Here's how the part is built. I have some questions about the finished solid (model axes, mm). Face numbers are marked on the shaded views. A direction names the side the tool comes from. Round coordinates to 2 decimals unless told otherwise and drop trailing zeros. Write each loop counter-clockwise with the first axis right and the second up, starting at its lowest first coordinate (ties: lowest second). Pieces come first, ordered by that corner, then holes. Notation, with made-up numbers: (11, 75.5) -> (15, 75.5) arc R25 cw to (15, 102.5) -> close; hole circle Ø10 at (-21.75, 44). An arc over 180 degrees is marked (long way). Answer in a Markdown table with one row per item. Add a question column.
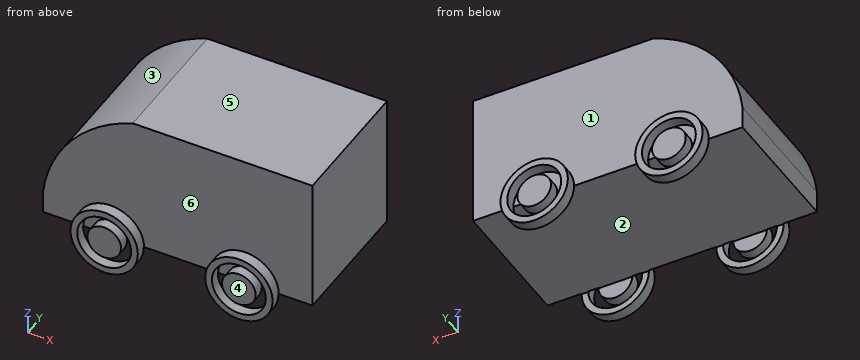
from build123d import *

# Parameters (mm, degrees)
F1_DEPTH = 76.2
F2_R     = 15.24
F3_DEPTH = 6.35
F2_R_2   = 9.525
F4_DEPTH = 6.35
F5_R     = 15.24
F6_DEPTH = 6.35
F5_R_2   = 9.525
F7_DEPTH = 6.35
F8_W     = 152.5372415781
F8_H     = 76.57238096
F9_DEPTH = 25.4


with BuildPart() as f1:
    # F0 (on Front) → F1 (new body)
    with BuildSketch(Plane.XZ):
        with BuildLine():
            Line((82.9111417405, 0), (101.9611417405, 0))
            Line((101.9611417405, 0), (101.9611417405, 76.2))
            Line((101.9611417405, 76.2), (0.3611417405, 76.2))
            ThreePointArc((0.3611417405, 76.2), (-34.2470067394, 51.816518784), (-50.4388582595, 12.7))
            Line((-50.4388582595, 12.7), (-50.4388582595, 0))
            Line((-50.4388582595, 0), (-31.3888582595, 0))
            ThreePointArc((-31.3888582595, 0), (-12.3388582595, 19.05), (6.7111417405, 0))
            Line((6.7111417405, 0), (44.8111417405, 0))
            ThreePointArc((44.8111417405, 0), (63.8611417405, 19.05), (82.9111417405, 0))
        make_face()
        with BuildLine():
            ThreePointArc((44.8111417405, 0), (63.8611417405, -19.05), (82.9111417405, 0))
            Line((82.9111417405, 0), (63.8611417405, 0))
            Line((63.8611417405, 0), (44.8111417405, 0))
        make_face()
        with BuildLine():
            Line((63.8611417405, 0), (82.9111417405, 0))
            ThreePointArc((82.9111417405, 0), (63.8611417405, 19.05), (44.8111417405, 0))
            Line((44.8111417405, 0), (63.8611417405, 0))
        make_face()
        with BuildLine():
            Line((-12.3388582595, 0), (6.7111417405, 0))
            ThreePointArc((6.7111417405, 0), (-12.3388582595, 19.05), (-31.3888582595, 0))
            Line((-31.3888582595, 0), (-12.3388582595, 0))
        make_face()
        with BuildLine():
            ThreePointArc((-31.3888582595, 0), (-12.3388582595, -19.05), (6.7111417405, 0))
            Line((6.7111417405, 0), (-12.3388582595, 0))
            Line((-12.3388582595, 0), (-31.3888582595, 0))
        make_face()
    extrude(amount=F1_DEPTH)

    # F2 (on face) → F3 (join)
    with BuildSketch(Plane.XZ.offset(76.2)):
        with BuildLine():
            ThreePointArc((82.9111417405, 0), (63.8611417405, 19.05), (44.8111417405, 0))
            ThreePointArc((44.8111417405, 0), (63.8611417405, -19.05), (82.9111417405, 0))
        make_face()
        with Locations((63.8611417405, 0)):
            Circle(F2_R, mode=Mode.SUBTRACT)
        with BuildLine():
            ThreePointArc((-31.3888582595, 0), (-12.3388582595, -19.05), (6.7111417405, 0))
            ThreePointArc((6.7111417405, 0), (-12.3388582595, 19.05), (-31.3888582595, 0))
        make_face()
        with Locations((-12.3388582595, 0)):
            Circle(F2_R, mode=Mode.SUBTRACT)
    extrude(amount=F3_DEPTH)

    # F2 (on face) → F4 (join)
    with BuildSketch(Plane.XZ.offset(76.2)):
        with Locations((63.8611417405, 0)):
            Circle(F2_R_2)
        with Locations((-12.3388582595, 0)):
            Circle(F2_R_2)
    extrude(amount=F4_DEPTH)

    # F5 (on face) → F6 (join)
    with BuildSketch(Plane(origin=(0, 0, 0), x_dir=(-1, 0, 0), z_dir=(0, 1, 0))):
        with BuildLine():
            ThreePointArc((-82.9111417405, 0), (-63.8611417405, -19.05), (-44.8111417405, 0))
            ThreePointArc((-44.8111417405, 0), (-63.8611417405, 19.05), (-82.9111417405, 0))
        make_face()
        with Locations((-63.8611417405, 0)):
            Circle(F5_R, mode=Mode.SUBTRACT)
        with BuildLine():
            ThreePointArc((31.3888582595, 0), (12.3388582595, 19.05), (-6.7111417405, 0))
            ThreePointArc((-6.7111417405, 0), (12.3388582595, -19.05), (31.3888582595, 0))
        make_face()
        with Locations((12.3388582595, 0)):
            Circle(F5_R, mode=Mode.SUBTRACT)
    extrude(amount=F6_DEPTH)

    # F5 (on face) → F7 (join)
    with BuildSketch(Plane(origin=(0, 0, 0), x_dir=(-1, 0, 0), z_dir=(0, 1, 0))):
        with Locations((-63.8611417405, 0)):
            Circle(F5_R_2)
        with Locations((12.3388582595, 0)):
            Circle(F5_R_2)
    extrude(amount=F7_DEPTH)

    # F8 (on face) → F9 (cut)
    with BuildSketch(Plane(origin=(0, 0, 0), x_dir=(1, 0, 0), z_dir=(0, 0, -1))):
        with Locations((25.47326684, 38.28619048)):
            Rectangle(F8_W, F8_H)
    extrude(amount=F9_DEPTH, mode=Mode.SUBTRACT)


solid = f1.part
Item 1: If we section it at A-A on x = 65: Please give me the cut outline in (y, z), then the cut area to 3 significant figures.
Item 2: If we section it at D-D on x = 16: Please give me the cut outline in (y, z).
Item 3: For P1, Ø3, axis at x = 71.5, z = 41, coming from the +Y side; P2, Ø5.5, axis at x = -18, z = -8, coming from the -Y side; P3, Ø1, axis at x = -9.5, z = 24.5, coming from the -Y side; P4, Ø12, axis at y = -27, z = 56, coming from the -X side, each with a flat end and sliding along its axis, tell me the tip position at first contact or that it passes through.
Item 4: If we section it at C-C on x = -4.5: Please give me the cut outline in (y, z), then the cut area to 3 significant figures.
Item 5: On a 3-axis mill with a long thin cutter (end or side, diameter ignored), from which of +Z, -Z, +X, -X, +Y, -Y can I reach the whole of each face in a straight line? I mean the marked faces 5 and 6. Say none if no direction works.
Item 6: If we mould it in two halves opening along Y, with no side actions, what happens to the marked faces 1, 2, 3 and 4? For each: pulls with the +Y half, pulls with the -Y half, needs draft (parallel to the pull), parting line crosses it, or undercut.
Item 7: If we section it at B-B on y = -36: Please give me the cut outline in (x, z).
Item 8: I need wall thicknesses on line 1 along Y through (x, z) = (29, 35); line 2 along Z through (x, y) = (6, -48.5); line 3 along Z through (x, y) = (-25, -5.5). Which ranges of each line are inside material? Lowest first, please. Write a range as from..to.
Results list:
| question | item | result |
|---|---|---|
| 1 | outline | (-82.55, -19.02) -> (-76.57, -19.02) -> (-76.57, -15.2) -> (-82.55, -15.2) -> close; (-82.55, -9.46) -> (-76.57, -9.46) -> (-76.57, 0) -> (0, 0) -> (0, -9.46) -> (6.35, -9.46) -> (6.35, 9.46) -> (0, 9.46) -> (0, 15.2) -> (6.35, 15.2) -> (6.35, 19.02) -> (0, 19.02) -> (0, 76.2) -> (-76.2, 76.2) -> (-76.2, 19.02) -> (-82.55, 19.02) -> (-82.55, 15.2) -> (-76.2, 15.2) -> (-76.2, 9.46) -> (-82.55, 9.46) -> close; (0, -19.02) -> (6.35, -19.02) -> (6.35, -15.2) -> (0, -15.2) -> close |
| 1 | area | 6,140 mm² |
| 2 | outline | (-76.2, 0) -> (0, 0) -> (0, 76.2) -> (-76.2, 76.2) -> close |
| 3 | P1 | y = 0 |
| 3 | P2 | y = -82.55 |
| 3 | P3 | y = -76.2 |
| 3 | P4 | x = -35.66 |
| 4 | outline | (-82.55, -17.36) -> (-76.57, -17.36) -> (-76.57, -13.07) -> (-82.55, -13.07) -> close; (-82.55, -5.41) -> (-76.57, -5.41) -> (-76.57, 0) -> (0, 0) -> (0, -5.41) -> (6.35, -5.41) -> (6.35, 5.41) -> (0, 5.41) -> (0, 13.07) -> (6.35, 13.07) -> (6.35, 17.36) -> (0, 17.36) -> (0, 74.34) -> (-76.2, 74.34) -> (-76.2, 17.36) -> (-82.55, 17.36) -> (-82.55, 13.07) -> (-76.2, 13.07) -> (-76.2, 5.41) -> (-82.55, 5.41) -> close; (0, -17.36) -> (6.35, -17.36) -> (6.35, -13.07) -> (0, -13.07) -> close |
| 4 | area | 5,910 mm² |
| 5 | face 5 | +Z, +X, -X, +Y, -Y |
| 5 | face 6 | +Z, -Y |
| 6 | face 1 | pulls with the +Y half |
| 6 | face 2 | undercut |
| 6 | face 3 | needs draft |
| 6 | face 4 | pulls with the -Y half |
| 7 | outline | (-50.44, 0) -> (101.96, 0) -> (101.96, 76.2) -> (0.36, 76.2) arc R75.99 ccw to (-50.44, 12.7) -> close |
| 8 | line 1 | -76.2..0 |
| 8 | line 2 | 0..76.2 |
| 8 | line 3 | 0..61.49 |
